```python
from build123d import *

# Parameters (mm, degrees)
BOSS_EXTRUDE1_DEPTH = 15
SKETCH3_R           = 3.05
CUT_EXTRUDE1_DEPTH  = 15
CUT_EXTRUDE3_DEPTH  = 59.485528143
SKETCH5_W           = 12.5375
SKETCH5_H           = 15
BOSS_EXTRUDE2_DEPTH = 1
CHAMFER1_SIZE       = 1
SKETCH6_W           = 40
SKETCH6_H           = 37
BOSS_EXTRUDE3_DEPTH = 5
CHAMFER2_SIZE       = 10


# Some blends are built 0.0001 mm under size
with BuildPart() as part:
    # Sketch2 → Boss-Extrude1 (new body)
    with BuildSketch(Plane(origin=(0, 0, 0), x_dir=(1, 0, 0), z_dir=(0, 1, 0))):
        Polygon((-13.5, 0), (6.5, 0), (11.5, -5), (11.5, -41), (31.917309801, -41), (31.917309801, -35.69895288), (16.5, -35.69895288), (16.5, 5), (-23.5, 5), (-23.5, -35.69895288), (-38.917309801, -35.69895288), (-38.917309801, -41), (-18.5, -41), (-18.5, -5), align=None)
    extrude(amount=BOSS_EXTRUDE1_DEPTH)

    # Sketch3 → Cut-Extrude1 (cut)
    with BuildSketch(Plane(origin=(0, 0, 35.69895288), x_dir=(-1, 0, 0), z_dir=(0, 0, -1))):
        with Locations((26.5, 9)):
            Circle(SKETCH3_R)
        with Locations((-23.5, 9)):
            Circle(SKETCH3_R)
    extrude(amount=-CUT_EXTRUDE1_DEPTH, mode=Mode.SUBTRACT)

    # Sketch4 → Cut-Extrude3 (cut, through all)
    with BuildSketch(Plane(origin=(0, 15, 0), x_dir=(1, 0, 0), z_dir=(0, 1, 0))):
        Polygon((-22, -10.075), (-20.075, -10.075), (-22, -12), (-22, -12.075), (-20.075, -12.075), (-22, -14), (-22, -14.075), (-20.075, -14.075), (-22, -16), (-22, -16.075), (-20.075, -16.075), (-22, -18), (-22, -18.075), (-20.075, -18.075), (-22, -20), (-22, -20.075), (-23.5, -20.075), (-23.5, -35.69895288), (-38.917309801, -35.69895288), (-38.917309801, -41), (-18.5, -41), (-18.5, -16.075), (-18.5, -8), (-20, -8), (-22, -10), align=None)
        Polygon((13, -8), (11.5, -8), (11.5, -41), (31.917309801, -41), (31.917309801, -35.69895288), (16.5, -35.69895288), (16.5, -20.075), (15, -20.075), (15, -20), (13.075, -18.075), (15, -18.075), (15, -18), (13.075, -16.075), (15, -16.075), (15, -16), (13.075, -14.075), (15, -14.075), (15, -14), (13.075, -12.075), (15, -12.075), (15, -12), (13.075, -10.075), (15, -10.075), (15, -10), align=None)
    extrude(amount=-CUT_EXTRUDE3_DEPTH, mode=Mode.SUBTRACT)

    # Sketch5 → Boss-Extrude2 (add)
    with BuildSketch(Plane.ZY.offset(23.5)):
        with Locations((13.80625, 7.5)):
            Rectangle(SKETCH5_W, SKETCH5_H)
    boss_extrude2 = extrude(amount=BOSS_EXTRUDE2_DEPTH)

    # Mirror1: Boss-Extrude2 across plane
    add(boss_extrude2.mirror(Plane(origin=(-3.5, 0, 0), x_dir=(0, 0, 1), z_dir=(1, 0, 0))))

    # Chamfer1
    chamfer1_edges = [part.edges().sort_by_distance(p)[0] for p in [
        (16.5, 7.5, 7.5375),
        (-23.5, 7.5, 7.5375),
    ]]
    chamfer(chamfer1_edges, length=CHAMFER1_SIZE - 0.0001)  # a hair under: the kernel refuses the full size

    # Sketch6 → Boss-Extrude3 (add)
    with BuildSketch(Plane(origin=(0, 0, -5), x_dir=(-1, 0, 0), z_dir=(0, 0, -1))):
        with Locations((3.5, 18.5)):
            Rectangle(SKETCH6_W, SKETCH6_H)
    extrude(amount=-BOSS_EXTRUDE3_DEPTH)

    # Chamfer2
    # the kernel refuses this chamfer: 10 mm, written as the material it adds along each edge
    with BuildSketch(Plane(origin=(42.21682988, 15, 0), x_dir=(0, -0.027495876610586317, 0.9996219169112968), z_dir=(-1, 0, 0))) as chamfer2_piece_1_section:
        Polygon((CHAMFER2_SIZE * 0.999621916911, CHAMFER2_SIZE * 0.0274958766106), (-CHAMFER2_SIZE * 0.0274958766106, CHAMFER2_SIZE * 0.999621916911), (0, 0), align=None)
    chamfer2_piece_1 = extrude(amount=61.433659759, mode=Mode.PRIVATE)
    chamfer2_piece_1 = split(chamfer2_piece_1, bisect_by=Plane(origin=(15.01875, 16.231233333, 10.01875), z_dir=(0.7071067811865479, 0, -0.7071067811865472)), keep=Keep.TOP, mode=Mode.PRIVATE)
    chamfer2_piece_1 = split(chamfer2_piece_1, bisect_by=Plane(origin=(17.5, 16.231233333, 7.537533333), z_dir=(-1, 0, 0)), keep=Keep.TOP, mode=Mode.PRIVATE)
    chamfer2_piece_1 = split(chamfer2_piece_1, bisect_by=Plane(origin=(17.499966667, 16.231233333, 7.5375), z_dir=(0, 0, 1)), keep=Keep.TOP, mode=Mode.PRIVATE)
    with BuildSketch(Plane(origin=(16.5, 15, 0), x_dir=(0, -0.027495876610586317, 0.9996219169112968), z_dir=(-1, 0, 0))) as chamfer2_piece_2_section:
        Polygon((CHAMFER2_SIZE * 0.999621916911, CHAMFER2_SIZE * 0.0274958766106), (-CHAMFER2_SIZE * 0.0274958766106, CHAMFER2_SIZE * 0.999621916911), (0, 0), align=None)
    chamfer2_piece_2 = extrude(amount=35.71682988, mode=Mode.PRIVATE)
    chamfer2_piece_2 = split(chamfer2_piece_2, bisect_by=Plane(origin=(15.769248019, 18.74844553, 8), z_dir=(0, 0, -1)), keep=Keep.TOP, mode=Mode.PRIVATE)
    chamfer2_piece_2 = split(chamfer2_piece_2, bisect_by=Plane(origin=(11.5, 18.74844553, 2.503108939), z_dir=(1, 0, 0)), keep=Keep.TOP, mode=Mode.PRIVATE)
    with BuildSketch(Plane(origin=(42.21682988, 15, 0), x_dir=(0, -0.027495876610586317, 0.9996219169112968), z_dir=(-1, 0, 0))) as chamfer2_piece_3_section:
        Polygon((CHAMFER2_SIZE * 0.999621916911, CHAMFER2_SIZE * 0.0274958766106), (-CHAMFER2_SIZE * 0.0274958766106, CHAMFER2_SIZE * 0.999621916911), (0, 0), align=None)
    chamfer2_piece_3 = extrude(amount=61.433659759, mode=Mode.PRIVATE)
    chamfer2_piece_3 = split(chamfer2_piece_3, bisect_by=Plane(origin=(16.985049673, 16.407833551, 7.022649673), z_dir=(-0.7071067811865476, 0, 0.7071067811865476)), keep=Keep.TOP, mode=Mode.PRIVATE)
    chamfer2_piece_3 = split(chamfer2_piece_3, bisect_by=Plane(origin=(15.253849673, 16.407833551, 8.753849673), z_dir=(0.7071067811865476, 0, -0.7071067811865476)), keep=Keep.TOP, mode=Mode.PRIVATE)
    chamfer2_piece_3 = split(chamfer2_piece_3, bisect_by=Plane(origin=(17.5, 16.407833551, 7.184332898), z_dir=(-1, 0, 0)), keep=Keep.TOP, mode=Mode.PRIVATE)
    with BuildSketch(Plane(origin=(42.21682988, 15, 0), x_dir=(0, -0.027495876610586317, 0.9996219169112968), z_dir=(-1, 0, 0))) as chamfer2_piece_4_section:
        Polygon((CHAMFER2_SIZE * 0.999621916911, CHAMFER2_SIZE * 0.0274958766106), (-CHAMFER2_SIZE * 0.0274958766106, CHAMFER2_SIZE * 0.999621916911), (0, 0), align=None)
    chamfer2_piece_4 = extrude(amount=61.433659759, mode=Mode.PRIVATE)
    chamfer2_piece_4 = split(chamfer2_piece_4, bisect_by=Plane(origin=(8.989616943, 19.750655371, 2.489616943), z_dir=(0.7071067811865476, 0, -0.7071067811865476)), keep=Keep.TOP, mode=Mode.PRIVATE)
    chamfer2_piece_4 = split(chamfer2_piece_4, bisect_by=Plane(origin=(15, 19.750655371, 0.498689257), z_dir=(-1, 0, 0)), keep=Keep.TOP, mode=Mode.PRIVATE)
    with BuildSketch(Plane(origin=(42.21682988, 15, 0), x_dir=(0, -0.027495876610586317, 0.9996219169112968), z_dir=(-1, 0, 0))) as chamfer2_piece_5_section:
        Polygon((CHAMFER2_SIZE * 0.999621916911, CHAMFER2_SIZE * 0.0274958766106), (-CHAMFER2_SIZE * 0.0274958766106, CHAMFER2_SIZE * 0.999621916911), (0, 0), align=None)
    chamfer2_piece_5 = extrude(amount=61.433659759, mode=Mode.PRIVATE)
    chamfer2_piece_5 = split(chamfer2_piece_5, bisect_by=Plane(origin=(-18.5, 16.119619514, 7.760760971), z_dir=(-1, 0, 0)), keep=Keep.TOP, mode=Mode.PRIVATE)
    chamfer2_piece_5 = split(chamfer2_piece_5, bisect_by=Plane(origin=(-18.85841494, 16.119619514, 8), z_dir=(0, 0, -1)), keep=Keep.TOP, mode=Mode.PRIVATE)
    with BuildSketch(Plane(origin=(42.21682988, 15, 0), x_dir=(0, -0.027495876610586317, 0.9996219169112968), z_dir=(-1, 0, 0))) as chamfer2_piece_6_section:
        Polygon((CHAMFER2_SIZE * 0.999621916911, CHAMFER2_SIZE * 0.0274958766106), (-CHAMFER2_SIZE * 0.0274958766106, CHAMFER2_SIZE * 0.999621916911), (0, 0), align=None)
    chamfer2_piece_6 = extrude(amount=61.433659759, mode=Mode.PRIVATE)
    chamfer2_piece_6 = split(chamfer2_piece_6, bisect_by=Plane(origin=(-15.875, 19.25, 2.375), z_dir=(-0.7071067811865475, 0, -0.7071067811865477)), keep=Keep.TOP, mode=Mode.PRIVATE)
    with BuildSketch(Plane(origin=(12.21682988, 15, 0), x_dir=(0, -0.027495876610586317, 0.9996219169112968), z_dir=(-1, 0, 0))) as chamfer2_piece_7_section:
        Polygon((CHAMFER2_SIZE * 0.999621916911, CHAMFER2_SIZE * 0.0274958766106), (-CHAMFER2_SIZE * 0.0274958766106, CHAMFER2_SIZE * 0.999621916911), (0, 0), align=None)
    chamfer2_piece_7 = extrude(amount=61.433659759, mode=Mode.PRIVATE)
    chamfer2_piece_7 = split(chamfer2_piece_7, bisect_by=Plane(origin=(11.85841494, 16.119619514, 8), z_dir=(0, 0, -1)), keep=Keep.TOP, mode=Mode.PRIVATE)
    chamfer2_piece_7 = split(chamfer2_piece_7, bisect_by=Plane(origin=(11.5, 16.119619514, 7.760760971), z_dir=(1, 0, 0)), keep=Keep.TOP, mode=Mode.PRIVATE)
    with BuildSketch(Plane(origin=(12.21682988, 15, 0), x_dir=(0, -0.027495876610586317, 0.9996219169112968), z_dir=(-1, 0, 0))) as chamfer2_piece_8_section:
        Polygon((CHAMFER2_SIZE * 0.999621916911, CHAMFER2_SIZE * 0.0274958766106), (-CHAMFER2_SIZE * 0.0274958766106, CHAMFER2_SIZE * 0.999621916911), (0, 0), align=None)
    chamfer2_piece_8 = extrude(amount=35.71682988, mode=Mode.PRIVATE)
    chamfer2_piece_8 = split(chamfer2_piece_8, bisect_by=Plane(origin=(-18.5, 16.112575477, 7.774849047), z_dir=(-1, 0, 0)), keep=Keep.TOP, mode=Mode.PRIVATE)
    chamfer2_piece_8 = split(chamfer2_piece_8, bisect_by=Plane(origin=(-19.137424523, 16.112575477, 8), z_dir=(0, 0, -1)), keep=Keep.TOP, mode=Mode.PRIVATE)
    with BuildSketch(Plane(origin=(12.21682988, 15, 0), x_dir=(0, -0.027495876610586317, 0.9996219169112968), z_dir=(-1, 0, 0))) as chamfer2_piece_9_section:
        Polygon((CHAMFER2_SIZE * 0.999621916911, CHAMFER2_SIZE * 0.0274958766106), (-CHAMFER2_SIZE * 0.0274958766106, CHAMFER2_SIZE * 0.999621916911), (0, 0), align=None)
    chamfer2_piece_9 = extrude(amount=61.433659759, mode=Mode.PRIVATE)
    chamfer2_piece_9 = split(chamfer2_piece_9, bisect_by=Plane(origin=(-18.5, 15.733974359, 8.532051282), z_dir=(-1, 0, 0)), keep=Keep.TOP, mode=Mode.PRIVATE)
    chamfer2_piece_9 = split(chamfer2_piece_9, bisect_by=Plane(origin=(-20.863782051, 15.733974359, 8.863782051), z_dir=(-0.7071067811865476, 0, -0.7071067811865476)), keep=Keep.TOP, mode=Mode.PRIVATE)
    chamfer2_piece_9 = split(chamfer2_piece_9, bisect_by=Plane(origin=(-24.5, 15.733974359, 8.532051282), z_dir=(1, 0, 0)), keep=Keep.TOP, mode=Mode.PRIVATE)
    chamfer2_piece_9 = split(chamfer2_piece_9, bisect_by=Plane(origin=(-23.344982051, 15.733974359, 6.382582051), z_dir=(0.7071067811865476, 0, 0.7071067811865476)), keep=Keep.TOP, mode=Mode.PRIVATE)
    with BuildSketch(Plane(origin=(12.21682988, 15, 0), x_dir=(0, -0.027495876610586317, 0.9996219169112968), z_dir=(-1, 0, 0))) as chamfer2_piece_10_section:
        Polygon((CHAMFER2_SIZE * 0.999621916911, CHAMFER2_SIZE * 0.0274958766106), (-CHAMFER2_SIZE * 0.0274958766106, CHAMFER2_SIZE * 0.999621916911), (0, 0), align=None)
    chamfer2_piece_10 = extrude(amount=61.433659759, mode=Mode.PRIVATE)
    chamfer2_piece_10 = split(chamfer2_piece_10, bisect_by=Plane(origin=(8.875, 19.25, 2.375), z_dir=(0.7071067811865476, 0, -0.7071067811865476)), keep=Keep.TOP, mode=Mode.PRIVATE)
    with BuildSketch(Plane(origin=(12.21682988, 15, 0), x_dir=(0, -0.027495876610586317, 0.9996219169112968), z_dir=(-1, 0, 0))) as chamfer2_piece_11_section:
        Polygon((CHAMFER2_SIZE * 0.999621916911, CHAMFER2_SIZE * 0.0274958766106), (-CHAMFER2_SIZE * 0.0274958766106, CHAMFER2_SIZE * 0.999621916911), (0, 0), align=None)
    chamfer2_piece_11 = extrude(amount=35.71682988, mode=Mode.PRIVATE)
    chamfer2_piece_11 = split(chamfer2_piece_11, bisect_by=Plane(origin=(-15.86117072, 19.18959267, 2.36117072), z_dir=(-0.7071067811865475, 0, -0.7071067811865477)), keep=Keep.TOP, mode=Mode.PRIVATE)
    with BuildSketch(Plane(origin=(12.21682988, 15, 0), x_dir=(0, -0.027495876610586317, 0.9996219169112968), z_dir=(-1, 0, 0))) as chamfer2_piece_12_section:
        Polygon((CHAMFER2_SIZE * 0.999621916911, CHAMFER2_SIZE * 0.0274958766106), (-CHAMFER2_SIZE * 0.0274958766106, CHAMFER2_SIZE * 0.999621916911), (0, 0), align=None)
    chamfer2_piece_12 = extrude(amount=61.433659759, mode=Mode.PRIVATE)
    chamfer2_piece_12 = split(chamfer2_piece_12, bisect_by=Plane(origin=(-24.5, 16.231233333, 7.537533333), z_dir=(1, 0, 0)), keep=Keep.TOP, mode=Mode.PRIVATE)
    chamfer2_piece_12 = split(chamfer2_piece_12, bisect_by=Plane(origin=(-24.499966667, 16.231233333, 7.5375), z_dir=(0, 0, 1)), keep=Keep.TOP, mode=Mode.PRIVATE)
    chamfer2_piece_12 = split(chamfer2_piece_12, bisect_by=Plane(origin=(-23.5, 16.231233333, 7.537533333), z_dir=(-1, 0, 0)), keep=Keep.TOP, mode=Mode.PRIVATE)
    add([chamfer2_piece_1, chamfer2_piece_2, chamfer2_piece_3, chamfer2_piece_4, chamfer2_piece_5, chamfer2_piece_6, chamfer2_piece_7, chamfer2_piece_8, chamfer2_piece_9, chamfer2_piece_10, chamfer2_piece_11, chamfer2_piece_12])


solid = part.part
```
Build history of the part. All positions in model axes, mm. A direction names the side the tool comes from. Round coordinates to 2 decimals unless told otherwise and drop trailing zeros. Write each loop counter-clockwise with the first axis right and the second up, starting at its lowest first coordinate (ties: lowest second). Pieces come first, ordered by that corner, then holes.
1) Drill centre lines: probe 1 along Z at (x, y) = (14, 13) (3 decimals); probe 2 along Z at (x, y) = (6, 34); probe 3 along X at (y, z) = (7.5, 16). Where is each one in solid material? Low to high.
2) Band-saw the part on C-C, the plane z = 0.75. List the corners of the cut face in (x, y), and give its area (3 significant figures).
3) Mould opens along X. For faces 1 (the flat face through (17.5, 9, 14)), 2 (the flat face through (14, 8, 19)), 3 (the flat face through (-20, 21, 4)) say: +X half, -X half, draft (parallel to the pull), parting line (faces both ways), or undercut.
4) Band-saw the part on A-A, the plane z = 15.5. List the corners of the cut face in (x, y), and give its area (3 significant figures).
5) Pin check, flat tips, straight feed: pin 1 (2 mm diameter, centred on x = 4, y = 20, fed in from +Z); pin 2 (9 mm diameter, centred on y = 10.5, z = 1.5, fed in from +X); pin 3 (1.3 mm diameter, centred on x = -21.5, z = 14.5, fed in from +Y); pin 4 (6 mm diameter, centred on x = -13.5, z = 0.5, fed in from -Y). Stop position of each tip, or through.
6) 3-axis set-ups, long thin cutter, end or side, ignore diameter. For faces 4 (the flat face through (-21, 8, 11)), 5 (the flat face through (-23.99, 9.1, 7.03)), 6 (the flat face through (11.5, 10, 6)), 7 (the flat face through (-23, 15, 15)): which of +Z, -Z, +X, -X, +Y, -Y reach the whole face in a straight line?
7) Band-saw the part on B-B, the plane x = 14. List the corners of the cut face in (y, z) (3 decimals), and give its area (3 significant figures).
Ans:
1. probe 1: z = -5 to 9, 10.075 to 11, 12.075 to 13, 14.075 to 15, 16.075 to 17, 18.075 to 19
1. probe 2: z = -5 to 0
1. probe 3: x = -24.5 to -22, 15 to 17.5
2. outline: (-23.5, 0) - (-14.25, 0) - (-14.25, 24.25) - (-23.5, 24.25) - close; (7.25, 0) - (16.5, 0) - (16.5, 24.25) - (7.25, 24.25) - close
2. area: 449 mm2
3. face 1: +X half
3. face 2: undercut
3. face 3: draft
4. outline: (-24.5, 0) - (-21.5, 0) - (-21.5, 15) - (-24.5, 15) - close; (14.5, 0) - (17.5, 0) - (17.5, 15) - (14.5, 15) - close
4. area: 90.0 mm2
5. pin 1: stops at z = 0
5. pin 2: stops at x = 16.5
5. pin 3: stops at y = 15
5. pin 4: stops at y = 0
6. face 4: +Y, -Y
6. face 5: -Z, -X, +Y, -Y
6. face 6: +Z, +Y, -Y
6. face 7: +Z, +X, -X, +Y
7. outline: (0, -5) - (37, -5) - (37, 0) - (25, 0) - (16, 9) - (0, 9) - close; (0, 10.075) - (15, 10.075) - (15, 11) - (0, 11) - close; (0, 12.075) - (15, 12.075) - (15, 13) - (0, 13) - close; (0, 14.075) - (15, 14.075) - (15, 15) - (0, 15) - close; (0, 16.075) - (15, 16.075) - (15, 17) - (0, 17) - close; (0, 18.075) - (15, 18.075) - (15, 19) - (0, 19) - close
7. area: 439 mm2
